from build123d import *

# Parameters (mm, degrees)
F0_R      = 22.5
F1_DEPTH  = 308.423
F4_DEPTH  = 31
F5_R      = 2.5
F6_DEPTH  = 40
F7_DEPTH  = 30
F8_R      = 2.5
F9_DEPTH  = 30
F10_R     = 35
F11_DEPTH = 10
F13_R     = 35
F14_DEPTH = 5


with BuildPart() as f1:
    # F0 (on Top) → F1 (new body)
    with BuildSketch(Plane.XY):
        Circle(F0_R)
    extrude(amount=F1_DEPTH)

    # F3 (on face) → F4 (join)
    with BuildSketch(Plane(origin=(0, 0, 0), x_dir=(1, 0, 0), z_dir=(0, 0, -1))):
        with BuildLine():
            ThreePointArc((7.0710678119, 2.5), (7.3919891974, 1.2682648404), (7.5, 0))
            ThreePointArc((7.5, 0), (7.3919069765, -1.268743966), (7.0707436663, -2.500916633))
            Line((7.0707436663, -2.500916633), (9.7997435124, -2.5))
            Line((9.7997435124, -2.5), (9.7997435124, 0))
            Line((9.7997435124, 0), (9.7997435124, 2.5))
            Line((9.7997435124, 2.5), (7.0710678119, 2.5))
        make_face()
        with BuildLine():
            Line((2.5, -9.7997435124), (2.5, -7.0710678119))
            ThreePointArc((2.5, -7.0710678119), (-0.0004861292, -7.4999999842), (-2.500916633, -7.0707436663))
            Line((-2.500916633, -7.0707436663), (-2.5, -9.7997435124))
            Line((-2.5, -9.7997435124), (0, -9.7997435124))
            Line((0, -9.7997435124), (2.5, -9.7997435124))
        make_face()
        with BuildLine():
            ThreePointArc((-7.0710678119, -2.5), (-7.4999999842, 0.0004861292), (-7.0707436663, 2.500916633))
            Line((-7.0707436663, 2.500916633), (-9.7997435124, 2.5))
            Line((-9.7997435124, 2.5), (-9.7997435124, 0))
            Line((-9.7997435124, 0), (-9.7997435124, -2.5))
            Line((-9.7997435124, -2.5), (-7.0710678119, -2.5))
        make_face()
        with BuildLine():
            ThreePointArc((7.0707436663, -2.500916633), (7.3919069765, -1.268743966), (7.5, 0))
            ThreePointArc((7.5, 0), (7.3919891974, 1.2682648404), (7.0710678119, 2.5))
            ThreePointArc((7.0710678119, 2.5), (5.303644593, 5.3029571025), (2.500916633, 7.0707436663))
            ThreePointArc((2.500916633, 7.0707436663), (0.0004861292, 7.4999999842), (-2.5, 7.0710678119))
            ThreePointArc((-2.5, 7.0710678119), (-5.3029571025, 5.303644593), (-7.0707436663, 2.500916633))
            ThreePointArc((-7.0707436663, 2.500916633), (-7.4999999842, 0.0004861292), (-7.0710678119, -2.5))
            ThreePointArc((-7.0710678119, -2.5), (-5.303644593, -5.3029571025), (-2.500916633, -7.0707436663))
            ThreePointArc((-2.500916633, -7.0707436663), (-0.0004861292, -7.4999999842), (2.5, -7.0710678119))
            ThreePointArc((2.5, -7.0710678119), (5.3029571025, -5.303644593), (7.0707436663, -2.500916633))
        make_face()
        with BuildLine():
            ThreePointArc((-2.5, 7.0710678119), (0.0004861292, 7.4999999842), (2.500916633, 7.0707436663))
            Line((2.500916633, 7.0707436663), (2.5, 9.7997435124))
            Line((2.5, 9.7997435124), (0, 9.7997435124))
            Line((0, 9.7997435124), (-2.5, 9.7997435124))
            Line((-2.5, 9.7997435124), (-2.5, 7.0710678119))
        make_face()
    extrude(amount=F4_DEPTH)

    # F5 (on face) → F6 (cut)
    with BuildSketch(Plane(origin=(0, 0, -31), x_dir=(1, 0, 0), z_dir=(0, 0, -1))):
        Circle(F5_R)
    extrude(amount=-F6_DEPTH, mode=Mode.SUBTRACT)

    # F2 (on face) → F7 (join)
    with BuildSketch(Plane.XY.offset(308.423)):
        with BuildLine():
            ThreePointArc((7.0707436663, -2.500916633), (7.3919069765, -1.268743966), (7.5, 0))
            ThreePointArc((7.5, 0), (7.3919891974, 1.2682648404), (7.0710678119, 2.5))
            ThreePointArc((7.0710678119, 2.5), (5.303644593, 5.3029571025), (2.500916633, 7.0707436663))
            ThreePointArc((2.500916633, 7.0707436663), (0.0004861292, 7.4999999842), (-2.5, 7.0710678119))
            ThreePointArc((-2.5, 7.0710678119), (-5.3029571025, 5.303644593), (-7.0707436663, 2.500916633))
            ThreePointArc((-7.0707436663, 2.500916633), (-7.4999999842, 0.0004861292), (-7.0710678119, -2.5))
            ThreePointArc((-7.0710678119, -2.5), (-5.303644593, -5.3029571025), (-2.500916633, -7.0707436663))
            ThreePointArc((-2.500916633, -7.0707436663), (-0.0004861292, -7.4999999842), (2.5, -7.0710678119))
            ThreePointArc((2.5, -7.0710678119), (5.3029571025, -5.303644593), (7.0707436663, -2.500916633))
        make_face()
        with BuildLine():
            ThreePointArc((-7.0710678119, -2.5), (-7.4999999842, 0.0004861292), (-7.0707436663, 2.500916633))
            Line((-7.0707436663, 2.500916633), (-9.7997435124, 2.5))
            Line((-9.7997435124, 2.5), (-9.7997435124, 0))
            Line((-9.7997435124, 0), (-9.7997435124, -2.5))
            Line((-9.7997435124, -2.5), (-7.0710678119, -2.5))
        make_face()
        with BuildLine():
            ThreePointArc((-2.5, 7.0710678119), (0.0004861292, 7.4999999842), (2.500916633, 7.0707436663))
            Line((2.500916633, 7.0707436663), (2.5, 9.7997435124))
            Line((2.5, 9.7997435124), (0, 9.7997435124))
            Line((0, 9.7997435124), (-2.5, 9.7997435124))
            Line((-2.5, 9.7997435124), (-2.5, 7.0710678119))
        make_face()
        with BuildLine():
            ThreePointArc((7.0710678119, 2.5), (7.3919891974, 1.2682648404), (7.5, 0))
            ThreePointArc((7.5, 0), (7.3919069765, -1.268743966), (7.0707436663, -2.500916633))
            Line((7.0707436663, -2.500916633), (9.7997435124, -2.5))
            Line((9.7997435124, -2.5), (9.7997435124, 0))
            Line((9.7997435124, 0), (9.7997435124, 2.5))
            Line((9.7997435124, 2.5), (7.0710678119, 2.5))
        make_face()
        with BuildLine():
            Line((2.5, -9.7997435124), (2.5, -7.0710678119))
            ThreePointArc((2.5, -7.0710678119), (-0.0004861292, -7.4999999842), (-2.500916633, -7.0707436663))
            Line((-2.500916633, -7.0707436663), (-2.5, -9.7997435124))
            Line((-2.5, -9.7997435124), (0, -9.7997435124))
            Line((0, -9.7997435124), (2.5, -9.7997435124))
        make_face()
    extrude(amount=F7_DEPTH)

    # F8 (on face) → F9 (cut)
    with BuildSketch(Plane.XY.offset(338.423)):
        Circle(F8_R)
    extrude(amount=-F9_DEPTH, mode=Mode.SUBTRACT)

    # F10 (on face) → F11 (join)
    with BuildSketch(Plane.XY.offset(308.423)):
        Circle(F10_R)
    extrude(amount=-F11_DEPTH)

    # F13 (on offset) → F14 (join)
    with BuildSketch(Plane.XY.offset(115)):
        Circle(F13_R)
    extrude(amount=F14_DEPTH)


solid = f1.part
Geometry: final body of the model. Coordinates: model frame, mm. A direction names the side the tool comes from. Coordinates: 2 decimals unless noted, no trailing zeros. Order: outer loops, then holes, each group sorted by start corner. A loop starts at its lowest first (then second) coordinate and runs counter-clockwise, first axis right, second up. Notation, with made-up numbers: (52, 28) - (67, 28) arc R16 ccw to (67, 56) - close; hole circle Ø3 at (86.5, -38). An arc over 180 degrees is marked (long way). Use one line per item in the form item = value.
1) Set-up query: faces 5 (the face through (0, -23, 298.423)), 6 (the face through (-28, -21, 303)), 7 (the face through (0, -23, 115)). Return all of +Z, -Z, +X, -X, +Y, -Y with unobstructed straight access to the full face (end or side cutting, diameter ignored); none if empty.
Solutions:
face_5 = none
face_6 = +Z, -Z
face_7 = -Z
2) Pin query (flat end, axial travel): pin 1 (0.8 mm diameter, centred on y = 8.5, z = -18, fed in from -X); pin 2 (1.5 mm diameter, centred on x = -4.5, z = 300.5, fed in from +Y); pin 3 (6 mm diameter, centred on x = -8, z = 265, fed in from -Y); pin 4 (4 mm diameter, centred on x = 26, z = 193.5, fed in from -Y). Return the tip coordinate at first contact, or that it passes through.
Solutions:
pin_1 = -2.5
pin_2 = 34.8
pin_3 = -21.94
pin_4 = through
3) Mould query, pull axis Z, two halves, no side actions, for faces 1 (the face through (0, -23, 120)), 2 (the face through (2, 2, 338.423)), 3 (the face through (-28, -21, 117)), 4 (the face through (10.382, -19.961, 207.963)). Classes: +Z half, -Z half, draft (parallel to the pull), parting line (faces both ways), or undercut.
Solutions:
face_1 = undercut
face_2 = +Z half
face_3 = draft
face_4 = undercut
4) Ray query, L1, parallel to Z at x = -12, y = -23; L2, parallel to Y at x = 0, z = 330. Return the intervals inside material, ascending.
Solutions:
L1 = 115 to 120, 298.42 to 308.42
L2 = -9.8 to -2.5, 2.5 to 9.8
5) Section A-A (x = 28). Return loops of the section in (y, z).
Solutions:
outline = (-21, 115) - (21, 115) - (21, 120) - (-21, 120) - close; (-21, 298.42) - (21, 298.42) - (21, 308.42) - (-21, 308.42) - close
6) Section B-B (z = 163.5). Return loops of the section in (x, y).
Solutions:
outline = circle Ø45 at (0, 0)
